Geometry check sheet. Reference: the model listing, model coordinates, mm. Face numbers are marked on the shaded views. A direction names the side the tool comes from. Give positions to 0.01 mm unless a question says otherwise; leave off trailing zeros. Order: outer loops, then holes, each group sorted by start corner. A loop starts at its lowest first (then second) coordinate and runs counter-clockwise, first axis right, second up. Notation, with made-up numbers: M 69.25,28 L 103.25,28 A29 ccw 103.25,65 Z; hole C 17,58 d2. An arc over 180 degrees is marked long. Answer as a JSON object with one key per item and string values. Group by question number.
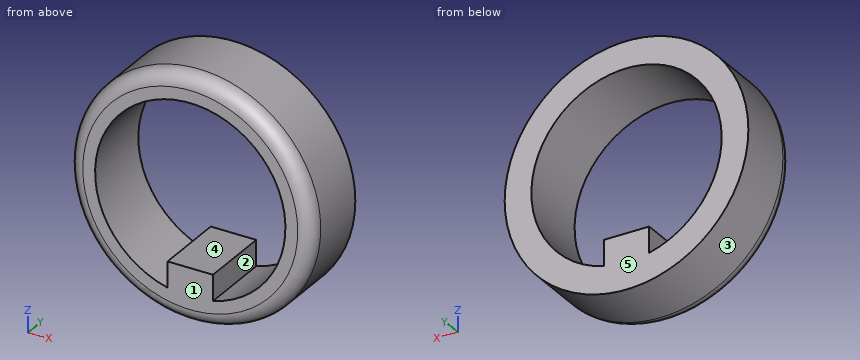
from build123d import *

# Parameters (mm, degrees)
SKETCH1_R           = 8.5
BOSS_EXTRUDE1_DEPTH = 5
FILLET3_R           = 1


with BuildPart() as part:
    # Sketch1 → Boss-Extrude1 (new body)
    with BuildSketch(Plane(origin=(0, 0, 0), x_dir=(1, 0, 0), z_dir=(0, 1, 0))):
        Circle(SKETCH1_R)
        with BuildLine():
            Line((-1.585, 6.447022258), (-1.585, 4.647022258))
            Line((-1.585, 4.647022258), (1.585, 4.647022258))
            Line((1.585, 4.647022258), (1.585, 6.447022258))
            ThreePointArc((1.585, 6.447022258), (0, -6.639), (-1.585, 6.447022258))
        make_face(mode=Mode.SUBTRACT)
    extrude(amount=BOSS_EXTRUDE1_DEPTH)

    # Fillet3
    fillet3_edges = [part.edges().sort_by_distance(p)[0] for p in [
        (-8.5, 0, 0),
    ]]
    fillet(fillet3_edges, radius=FILLET3_R)


solid = part.part
1. Release check for a two-part mould opening along Z. For the marked faces 3, 4 and 5 record: released by +Z, released by -Z, zero draft, split by the parting line, or undercut.
2. Thickness scan on line 1 along X through (y, z) = (1.95, 0); line 2 along X through (y, z) = (0.9, -5.25) (1 decimal); line 3 along X through (y, z) = (4.55, 4). Record the ranges inside material, lowest first. Write a range as [from, to].
3. Cross-section at B-B (x = 0). Record the cut outline in (y, z), and give its area (3 significant figures).
4. Depth check by flat-ended pin: pin 1 (2 mm diameter, centred on x = 6.5, y = 4, fed in from -Z); pin 2 (2 mm diameter, centred on y = 2, z = -5.5, fed in from -X); pin 3 (1.4 mm diameter, centred on y = 2.5, z = -5.5, fed in from +X) (3 decimals); pin 4 (10 mm diameter, centred on x = 5, z = -1.5, fed in from +Y). Enter the tip coordinate at first touch or a pass-through.
5. Cross-section at C-C (y = 3). Record the cut outline in (x, z) (3 decimals), and give its area (3 significant figures).
6. Access from +Z, -Z, +X, -X, +Y, -Y to the whole of each face (thin tool, end or side, straight path). Record for the marked faces 1 and 2.
7. Cross-section at A-A (z = 0). Record the cut outline in (x, y), and give its area (3 significant figures).
Report:
{
 "1": {"face 3": "split by the parting line", "face 4": "undercut", "face 5": "zero draft"},
 "2": {"line 1": "x = [-8.5, -6.64], [6.64, 8.5]", "line 2": "x = [-6.7, -4.1], [-1.6, 1.6], [4.1, 6.7]", "line 3": "x = [-7.5, -5.3], [5.3, 7.5]"},
 "3": {"outline": "M 0,-7.5 A1 ccw 1,-8.5 L 5,-8.5 L 5,-4.65 L 0,-4.65 Z; M 0,6.64 L 5,6.64 L 5,8.5 L 1,8.5 A1 ccw 0,7.5 Z", "area": "28.1 mm2"},
 "4": {"pin 1": "stops at z = -6.48", "pin 2": "stops at x = -7.21", "pin 3": "stops at x = 7.015", "pin 4": "stops at y = 5"},
 "5": {"outline": "C 0,0 d17; hole M -1.585,-6.447 L -1.585,-4.647 L 1.585,-4.647 L 1.585,-6.447 A6.639 ccw long Z", "area": "94.6 mm2"},
 "6": {"face 1": "+Z, -Z, +X, -X, -Y", "face 2": "+Y, -Y"},
 "7": {"outline": "M -8.5,1 A1 ccw -7.5,0 L -6.64,0 L -6.64,5 L -8.5,5 Z; M 6.64,0 L 7.5,0 A1 ccw 8.5,1 L 8.5,5 L 6.64,5 Z", "area": "18.2 mm2"}
}
